Autodesk Inventor part; units mm, degrees
ref_plane "bolt_XY" through (0, 0, 0) normal (1, 0, 0) x (0, 0, -1)
ref_plane "bolt_YZ" through (0, 0, 0) normal (0, 0, -1) x (0, 1, 0)
ref_plane "bolt_ZX" through (0, 0, 0) normal (0, 1, 0) x (1, 0, 0)
sketch "Sketch_1" plane through (0, 0, 0) normal (0, 0, 1) x (1, 0, 0)
  line L0 (18, 0) -> (-5, 0)
  line L1 (-5, 0) -> (-5, 4.25)
  line L2 (-5, 4.25) -> (0, 4.25)
  line L3 (0, 4.25) -> (0, 2.5)
  line L4 (0, 2.5) -> (17.5095, 2.5)
  line L5 (17.5095, 2.5) -> (18, 2.0095)
  line L6 (18, 2.0095) -> (18, 0)
  line L7 (18, 0) -> (-5, 0)
revolve "Revolution1" add sketch "Sketch_1" angle 360 about axis through (18, 0, 0) along (1, 0, 0)
thread "Thread1"
sketch "Sketch_4" plane through (0, 0, 0) normal (0, 0, 1) x (1, 0, 0)
  line L0 (-1.9641, 0) -> (-5, 0)
  line L1 (-5, 0) -> (-5, 2)
  line L2 (-5, 2) -> (-2.5, 2)
  line L3 (-2.5, 2) -> (-1.9641, 0)
  line L4 (-1.9641, 0) -> (-5, 0)
revolve "Revolution2" cut sketch "Sketch_4" angle 360 about axis through (-1.9641, 0, 0) along (1, 0, 0)
sketch "Sketch_3" plane through (-5, 0, 0) normal (1, 0, 0) x (0, 0, -1)
  line L0 (-2, 1.1547) -> (-2, -1.1547)
  line L1 (-2, -1.1547) -> (0, -2.3094)
  line L2 (0, -2.3094) -> (2, -1.1547)
  line L3 (2, -1.1547) -> (2, 1.1547)
  line L4 (2, 1.1547) -> (0, 2.3094)
  line L5 (0, 2.3094) -> (-2, 1.1547)
extrude "Extrusion1" cut sketch "Sketch_3" along normal blind 2.5
ref_plane "bolt_XY" through (0, 0, 0) normal (1, 0, 0) x (0, 0, -1)
ref_plane "bolt_YZ" through (0, 0, 0) normal (0, 0, -1) x (0, 1, 0)
ref_plane "bolt_ZX" through (0, 0, 0) normal (0, 1, 0) x (1, 0, 0)
ref_plane "nut_XY" through (18, 0, 0) normal (1, 0, 0) x (0, 0, -1)
ref_plane "nut_YZ" through (18, 0, 0) normal (0, 0, -1) x (0, 1, 0)
ref_plane "nut_ZX" through (18, 0, 0) normal (0, 1, 0) x (1, 0, 0)
properties part number "CBM5-18" material "MISUMI"
Work out the finished part from the listing and answer in its coordinate system (mm). A direction names the side the tool comes from. Give positions to 0.01 mm unless a question says otherwise; leave off trailing zeros. Write each loop counter-clockwise with the first axis right and the second up, starting at its lowest first coordinate (ties: lowest second). Pieces come first, ordered by that corner, then holes. Notation, with made-up numbers: (82, -30.75) - (102, -30.75) arc R26 cw to (102, 6.25) - close; hole circle Ø9 at (47, 73). An arc over 180 degrees is marked (long way). One line per item, written item: value. Start each with the question number.
1. Consider probe 1 along Z at (x, y) = (9, 1.5); probe 2 along X at (y, z) = (-1, -3). Determine where each line is inside the solid, lowest interval first.
2. For faces 4 (the flat face through (18, 0, 0)), 5 (the flat face through (-3.768, -1.724, 1.014)), 6 (the flat face through (0, 2, -2)), determine the directions among +Z, -Z, +X, -X, +Y, -Y from which every point of the face is accessible in a straight line to the end or side of a thin tool.
3. Given pin 1 (5 mm diameter, centred on x = 12.5, y = -2, fed in from -Z); pin 2 (0.5 mm diameter, centred on y = 0.5, z = -1.5, fed in from -X); pin 3 (3 mm diameter, centred on x = 5, z = 3, fed in from -Y), each flat-ended and moving along its own axis, determine where each tip first touches the part or whether it passes through.
4. For a pull along Y with two mould halves and no side action, classify faces 1 (the flat face through (-5, 2, -1)), 2 (the cylindrical face through (-2.465, 2.285, 3.584)), 3 (the flat face through (-3.77, -1.74, -0.99)) as +Y half, -Y half, draft (parallel to the pull), parting line (faces both ways), or undercut.
5. Find section A-A (x = 8). Write down the section's boundary in (y, z), then the cut area to 3 significant figures.
6. Find section B-B (z = -3.5). Write down the section's boundary in (x, y).
Geometry results:
1. probe 1: -2 to 2
1. probe 2: -5 to 0
2. face 4: +Z, -Z, +X, +Y, -Y
2. face 5: -X
2. face 6: +X
3. pin 1: z = -2.5
3. pin 2: x = -2.45
3. pin 3: y = -2
4. face 1: draft
4. face 2: parting line
4. face 3: undercut
5. outline: circle Ø5 at (0, 0)
5. area: 19.6 mm2
6. outline: (-5, -2.41) - (0, -2.41) - (0, 2.41) - (-5, 2.41) - close
